Read the model definition and answer for the solid it produces. Units are mm, in the model's axes. A direction names the side the tool comes from. Coordinates: 2 decimals unless noted, no trailing zeros. Write each loop counter-clockwise with the first axis right and the second up, starting at its lowest first coordinate (ties: lowest second). Pieces come first, ordered by that corner, then holes. Notation, with made-up numbers: (-27.75, 59.25) -> (8.25, 59.25) arc R23 cw to (8.25, 93.25) -> close; hole circle Ø8 at (24.25, 76.5). An arc over 180 degrees is marked (long way). One line per item, written item: value. Start each with the question number.
1. For a pull along Y with two mould halves and no side action, classify faces 1 (the flat face through (51.2, 22, 36)), 2 (the flat face through (-42, 37.5, 26)), 3 (the cylindrical face through (-8.964, -8.771, 2.535)), 4 (the flat face through (45.4, 23, 38)) as pulls with the +Y half, pulls with the -Y half, needs draft (parallel to the pull), parting line crosses it, or undercut.
2. Find section C-C, the plane y = 8.5. Write down the section's boundary in (x, z).
3. Consider line 1 along Y through (x, z) = (0, 1.65); line 2 along X through (y, z) = (27.5, 32); line 3 along Y through (x, z) = (-45, 63.5). Determine where each line is inside the solid, lowest interval first.
4. Find section D-D, the plane x = 54.5. Write down the section's boundary in (y, z).
5. For faces 5 (the flat face through (48, 27, 32)), 6 (the flat face through (42, 37.5, 26)), 7 (the flat face through (-43, 33.7, 38)), 8 (the cylindrical face through (0, 48, 3)), determine the directions among +Z, -Z, +X, -X, +Y, -Y from which every point of the face is accessible in a straight line to the end or side of a thin tool.
6. Find section B-B, the plane y = 30.5. Write down the section's boundary in (x, z), and give its area (3 significant figures).
7. Find section A-A, the plane z = 13.5. Write down the section's boundary in (x, y).
8. Given P1, Ø6, axis at x = 35, y = 32.5, coming from the +Z side; P2, Ø1.7, axis at x = -47, z = 59, coming from the -Y side; P3, Ø6.5, axis at x = -48.5, z = 32, coming from the +Y side; P4, Ø12, axis at x = -6.5, y = 20.5, coming from the -Z side, each flat-ended and moving along its own axis, determine where each tip first touches the part or whether it passes through.
```python
from build123d import *

# Parameters (mm, degrees)
BOX011_W                    = 6
BOX011_H                    = 4
BOX011_DEPTH                = 12
FILLET009_R                 = 1.9
BOX013_W                    = 4.2
BOX013_H                    = 17.4
BOX013_DEPTH                = 67
BOX010_W                    = 6
BOX010_H                    = 4
BOX010_DEPTH                = 12
FILLET008_R                 = 1.9
BOX012_W                    = 10
BOX012_H                    = 25
BOX012_DEPTH                = 67
BOX007_W                    = 4.2
BOX007_H                    = 17.4
BOX007_DEPTH                = 67
BOX008_W                    = 6
BOX008_H                    = 4
BOX008_DEPTH                = 12
FILLET006_R                 = 1.9
BOX009_W                    = 6
BOX009_H                    = 4
BOX009_DEPTH                = 12
FILLET007_R                 = 1.9
BOX006_W                    = 10
BOX006_H                    = 25
BOX006_DEPTH                = 67
CYLINDER002_W               = 66
CYLINDER002_H               = 5
CYLINDER002_ANGLE           = 15
CYLINDER002_PLACEMENT_ANGLE = 14.5
CYLINDER001_W               = 70
CYLINDER001_H               = 5
CYLINDER001_ANGLE           = 15
CYLINDER001_PLACEMENT_ANGLE = 14.5
CYLINDER004_W               = 48
CYLINDER004_H               = 5
CYLINDER004_ANGLE           = 15
CYLINDER004_PLACEMENT_ANGLE = 82.5
CYLINDER003_W               = 52
CYLINDER003_H               = 5
CYLINDER003_ANGLE           = 15
CYLINDER003_PLACEMENT_ANGLE = 82.5
CYLINDER007_R               = 2
CYLINDER007_DEPTH           = 5
CYLINDER006_W               = 66
CYLINDER006_H               = 5
CYLINDER006_ANGLE           = 15
CYLINDER006_PLACEMENT_ANGLE = 150.5
CYLINDER005_W               = 70
CYLINDER005_H               = 5
CYLINDER005_ANGLE           = 15
CYLINDER005_PLACEMENT_ANGLE = 150.5
BOX015_W                    = 25
BOX015_H                    = 75
BOX015_DEPTH                = 5
FILLET011_R                 = 12.4
BOX014_W                    = 152.4
BOX014_H                    = 25
BOX014_DEPTH                = 5
FILLET010_R                 = 12.4


with BuildPart() as fillet009:
    # Box011 → Box011 (new body)
    with BuildSketch(Plane(origin=(-45, 23, 26), x_dir=(1, 0, 0), z_dir=(0, 0, 1))):
        with Locations((3, 2)):
            Rectangle(BOX011_W, BOX011_H)
    extrude(amount=BOX011_DEPTH)

    # Fillet009
    fillet009_edges = [fillet009.edges().sort_by_distance(p)[0] for p in [
        (-42, 23, 26),
        (-42, 23, 38),
        (-42, 27, 26),
        (-42, 27, 38),
    ]]
    fillet(fillet009_edges, radius=FILLET009_R)


with BuildPart() as obj1:
    # Box013 → Box013 (new body)
    with BuildSketch(Plane(origin=(-39.2, 16.3, 10), x_dir=(1, 0, 0), z_dir=(0, 0, 1))):
        with Locations((2.1, 8.7)):
            Rectangle(BOX013_W, BOX013_H)
    extrude(amount=BOX013_DEPTH)


with BuildPart() as fusion003:
    # Box010 → Box010 (new body)
    with BuildSketch(Plane(origin=(-45, 23, 54), x_dir=(1, 0, 0), z_dir=(0, 0, 1))):
        with Locations((3, 2)):
            Rectangle(BOX010_W, BOX010_H)
    extrude(amount=BOX010_DEPTH)

    # Fillet008
    fillet008_edges = [fusion003.edges().sort_by_distance(p)[0] for p in [
        (-42, 23, 54),
        (-42, 23, 66),
        (-42, 27, 54),
        (-42, 27, 66),
    ]]
    fillet(fillet008_edges, radius=FILLET008_R)

    # Fusion003: union Fillet009, obj1
    add(fillet009.part)
    add(obj1.part)


with BuildPart() as stuetze002:
    # Box012 → Box012 (new body)
    with BuildSketch(Plane(origin=(-45, 12.5, 0), x_dir=(1, 0, 0), z_dir=(0, 0, 1))):
        with Locations((5, 12.5)):
            Rectangle(BOX012_W, BOX012_H)
    extrude(amount=BOX012_DEPTH)

    # Cut006: cut Fusion003
    add(fusion003.part, mode=Mode.SUBTRACT)


with BuildPart() as stuetze002_1:
    # Cut006 placement: moved
    add(stuetze002.part.moved(Location((-6.2, 0, 0))))


with BuildPart() as obj2:
    # Box007 → Box007 (new body)
    with BuildSketch(Plane(origin=(35, 16.3, 10), x_dir=(1, 0, 0), z_dir=(0, 0, 1))):
        with Locations((2.1, 8.7)):
            Rectangle(BOX007_W, BOX007_H)
    extrude(amount=BOX007_DEPTH)


with BuildPart() as fillet006:
    # Box008 → Box008 (new body)
    with BuildSketch(Plane(origin=(39, 23, 54), x_dir=(1, 0, 0), z_dir=(0, 0, 1))):
        with Locations((3, 2)):
            Rectangle(BOX008_W, BOX008_H)
    extrude(amount=BOX008_DEPTH)

    # Fillet006
    fillet006_edges = [fillet006.edges().sort_by_distance(p)[0] for p in [
        (42, 23, 54),
        (42, 23, 66),
        (42, 27, 54),
        (42, 27, 66),
    ]]
    fillet(fillet006_edges, radius=FILLET006_R)


with BuildPart() as fusion002:
    # Box009 → Box009 (new body)
    with BuildSketch(Plane(origin=(39, 23, 26), x_dir=(1, 0, 0), z_dir=(0, 0, 1))):
        with Locations((3, 2)):
            Rectangle(BOX009_W, BOX009_H)
    extrude(amount=BOX009_DEPTH)

    # Fillet007
    fillet007_edges = [fusion002.edges().sort_by_distance(p)[0] for p in [
        (42, 23, 26),
        (42, 23, 38),
        (42, 27, 26),
        (42, 27, 38),
    ]]
    fillet(fillet007_edges, radius=FILLET007_R)

    # Fusion002: union obj2, Fillet006
    add(obj2.part)
    add(fillet006.part)


with BuildPart() as stuetze001:
    # Box006 → Box006 (new body)
    with BuildSketch(Plane(origin=(35, 12.5, 0), x_dir=(1, 0, 0), z_dir=(0, 0, 1))):
        with Locations((5, 12.5)):
            Rectangle(BOX006_W, BOX006_H)
    extrude(amount=BOX006_DEPTH)

    # Cut005: cut Fusion002
    add(fusion002.part, mode=Mode.SUBTRACT)


with BuildPart() as stuetze001_1:
    # Cut005 placement: moved
    add(stuetze001.part.moved(Location((6.2, 0, 0))))


with BuildPart() as zylinder002:
    # Cylinder002 → Cylinder002 (revolve)
    with BuildSketch(Plane.XZ):
        with Locations((33, 2.5)):
            Rectangle(CYLINDER002_W, CYLINDER002_H)
    revolve(axis=Axis((0, 0, 0), (0, 0, 1)), revolution_arc=CYLINDER002_ANGLE)


with BuildPart() as zylinder002_1:
    # Cylinder002 placement: moved
    add(zylinder002.part.rotate(Axis((0, 0, 0), (0, 0, 1)), CYLINDER002_PLACEMENT_ANGLE))


with BuildPart() as obj3:
    # Cylinder001 → Cylinder001 (revolve)
    with BuildSketch(Plane.XZ):
        with Locations((35, 2.5)):
            Rectangle(CYLINDER001_W, CYLINDER001_H)
    revolve(axis=Axis((0, 0, 0), (0, 0, 1)), revolution_arc=CYLINDER001_ANGLE)


with BuildPart() as obj3_1:
    # Cylinder001 placement: moved
    add(obj3.part.rotate(Axis((0, 0, 0), (0, 0, 1)), CYLINDER001_PLACEMENT_ANGLE))

    # Cut: cut Zylinder002
    add(zylinder002_1.part, mode=Mode.SUBTRACT)


with BuildPart() as zylinder004:
    # Cylinder004 → Cylinder004 (revolve)
    with BuildSketch(Plane.XZ):
        with Locations((24, 2.5)):
            Rectangle(CYLINDER004_W, CYLINDER004_H)
    revolve(axis=Axis((0, 0, 0), (0, 0, 1)), revolution_arc=CYLINDER004_ANGLE)


with BuildPart() as zylinder004_1:
    # Cylinder004 placement: moved
    add(zylinder004.part.rotate(Axis((0, 0, 0), (0, 0, 1)), CYLINDER004_PLACEMENT_ANGLE))


with BuildPart() as obj4:
    # Cylinder003 → Cylinder003 (revolve)
    with BuildSketch(Plane.XZ):
        with Locations((26, 2.5)):
            Rectangle(CYLINDER003_W, CYLINDER003_H)
    revolve(axis=Axis((0, 0, 0), (0, 0, 1)), revolution_arc=CYLINDER003_ANGLE)


with BuildPart() as obj4_1:
    # Cylinder003 placement: moved
    add(obj4.part.rotate(Axis((0, 0, 0), (0, 0, 1)), CYLINDER003_PLACEMENT_ANGLE))

    # Cut001: cut Zylinder004
    add(zylinder004_1.part, mode=Mode.SUBTRACT)


with BuildPart() as obj5:
    # Cylinder007 → Cylinder007 (new body)
    with BuildSketch(Plane.XY):
        Circle(CYLINDER007_R)
    extrude(amount=CYLINDER007_DEPTH)


with BuildPart() as zylinder006:
    # Cylinder006 → Cylinder006 (revolve)
    with BuildSketch(Plane.XZ):
        with Locations((33, 2.5)):
            Rectangle(CYLINDER006_W, CYLINDER006_H)
    revolve(axis=Axis((0, 0, 0), (0, 0, 1)), revolution_arc=CYLINDER006_ANGLE)


with BuildPart() as zylinder006_1:
    # Cylinder006 placement: moved
    add(zylinder006.part.rotate(Axis((0, 0, 0), (0, 0, 1)), CYLINDER006_PLACEMENT_ANGLE))


with BuildPart() as obj6:
    # Cylinder005 → Cylinder005 (revolve)
    with BuildSketch(Plane.XZ):
        with Locations((35, 2.5)):
            Rectangle(CYLINDER005_W, CYLINDER005_H)
    revolve(axis=Axis((0, 0, 0), (0, 0, 1)), revolution_arc=CYLINDER005_ANGLE)


with BuildPart() as obj6_1:
    # Cylinder005 placement: moved
    add(obj6.part.rotate(Axis((0, 0, 0), (0, 0, 1)), CYLINDER005_PLACEMENT_ANGLE))

    # Cut002: cut Zylinder006
    add(zylinder006_1.part, mode=Mode.SUBTRACT)

    # Fusion004: union obj3, obj4, obj5
    add(obj3_1.part)
    add(obj4_1.part)
    add(obj5.part)


with BuildPart() as fillet002:
    # Box015 → Box015 (new body)
    with BuildSketch(Plane(origin=(-12.5, -12.5, 0), x_dir=(1, 0, 0), z_dir=(0, 0, 1))):
        with Locations((12.5, 37.5)):
            Rectangle(BOX015_W, BOX015_H)
    extrude(amount=BOX015_DEPTH)

    # Fillet011
    fillet011_edges = [fillet002.edges().sort_by_distance(p)[0] for p in [
        (-12.5, -12.5, 2.5),
        (-12.5, 62.5, 2.5),
        (12.5, -12.5, 2.5),
        (12.5, 62.5, 2.5),
    ]]
    fillet(fillet011_edges, radius=FILLET011_R)


with BuildPart() as fusion:
    # Box014 → Box014 (new body)
    with BuildSketch(Plane(origin=(-76.2, 12.5, 0), x_dir=(1, 0, 0), z_dir=(0, 0, 1))):
        with Locations((76.2, 12.5)):
            Rectangle(BOX014_W, BOX014_H)
    extrude(amount=BOX014_DEPTH)

    # Fillet010
    fillet010_edges = [fusion.edges().sort_by_distance(p)[0] for p in [
        (-76.2, 12.5, 2.5),
        (-76.2, 37.5, 2.5),
        (76.2, 12.5, 2.5),
        (76.2, 37.5, 2.5),
    ]]
    fillet(fillet010_edges, radius=FILLET010_R)

    # Fusion005: union Fillet002
    add(fillet002.part)

    # Cut007: cut obj6
    add(obj6_1.part, mode=Mode.SUBTRACT)

    # Fusion: union Stuetze002, Stuetze001
    add(stuetze002_1.part)
    add(stuetze001_1.part)


solid = fusion.part
```
Answer block:
1. face 1: needs draft
1. face 2: pulls with the +Y half
1. face 3: pulls with the -Y half
1. face 4: undercut
2. outline: (-12.5, 0) -> (12.5, 0) -> (12.5, 5) -> (-12.5, 5) -> close
3. line 1: y = -12.5 to -2, 2 to 48, 52 to 62.5
3. line 2: x = -51.2 to -45.4, 45.4 to 51.2
3. line 3: y = 12.5 to 16.3, 33.7 to 37.5
4. outline: (12.5, 0) -> (37.5, 0) -> (37.5, 5) -> (12.5, 5) -> close
5. face 5: +X, -X
5. face 6: +Z, -Z, +X, +Y
5. face 7: +Z
5. face 8: +Z, -Z
6. outline: (-74.96, 0) -> (-63.01, 0) -> (-63.01, 5) -> (-74.96, 5) -> close; (-58.53, 0) -> (58.53, 0) -> (58.53, 5) -> (51.2, 5) -> (51.2, 67) -> (45.4, 67) -> (45.4, 10) -> (41.2, 10) -> (41.2, 5) -> (-41.2, 5) -> (-41.2, 10) -> (-45.4, 10) -> (-45.4, 67) -> (-51.2, 67) -> (-51.2, 5) -> (-58.53, 5) -> close; (63.01, 0) -> (74.96, 0) -> (74.96, 5) -> (63.01, 5) -> close
6. area: 1,470 mm2
7. outline: (-51.2, 12.5) -> (-41.2, 12.5) -> (-41.2, 16.3) -> (-45.4, 16.3) -> (-45.4, 33.7) -> (-41.2, 33.7) -> (-41.2, 37.5) -> (-51.2, 37.5) -> close; (41.2, 12.5) -> (51.2, 12.5) -> (51.2, 37.5) -> (41.2, 37.5) -> (41.2, 33.7) -> (45.4, 33.7) -> (45.4, 16.3) -> (41.2, 16.3) -> close
8. P1: stops at z = 5
8. P2: stops at y = 12.5
8. P3: stops at y = 37.5
8. P4: stops at z = 0
